Check sheet for the modelled part. Datum: model origin and axes. Units: mm. Round coordinates to 2 decimals unless told otherwise and drop trailing zeros. Loops run counter-clockwise (first coordinate to the right, second up) from the corner with the lowest first, then second, coordinate; pieces in that order, holes last. Notation, with made-up numbers: (7, 48) - (26, 48) arc R18 cw to (26, 56) - close; hole circle Ø2 at (26, 27). An arc over 180 degrees is marked (long way). Return JSON: item names as keys, results as strings.
from build123d import *

# Parameters (mm, degrees)
TOP_PLATE_SKETCH_PROFILE_R   = 3.175
TOP_PLATE_SKETCH_PROFILE_R_2 = 2.69875
TOP_PLATE_EXTRUDE_DEPTH      = 12.7


with BuildPart() as part:
    # Top Plate Sketch Profile → Top Plate Extrude (new body)
    with BuildSketch(Plane.XY.offset(114.3)):
        with BuildLine():
            Line((50.8, 44.45), (50.8, -44.45))
            ThreePointArc((50.8, -44.45), (48.940128061, -48.940128061), (44.45, -50.8))
            Line((44.45, -50.8), (-44.45, -50.8))
            ThreePointArc((-44.45, -50.8), (-48.940128061, -48.940128061), (-50.8, -44.45))
            Line((-50.8, -44.45), (-50.8, 44.45))
            ThreePointArc((-50.8, 44.45), (-48.940128061, 48.940128061), (-44.45, 50.8))
            Line((-44.45, 50.8), (44.45, 50.8))
            ThreePointArc((44.45, 50.8), (48.940128061, 48.940128061), (50.8, 44.45))
        make_face()
        with Locations((42.8625, 0)):
            Circle(TOP_PLATE_SKETCH_PROFILE_R, mode=Mode.SUBTRACT)
        with Locations((-42.8625, 0)):
            Circle(TOP_PLATE_SKETCH_PROFILE_R, mode=Mode.SUBTRACT)
        with Locations((-42.8625, 42.8625)):
            Circle(TOP_PLATE_SKETCH_PROFILE_R_2, mode=Mode.SUBTRACT)
        with Locations((42.8625, 42.8625)):
            Circle(TOP_PLATE_SKETCH_PROFILE_R_2, mode=Mode.SUBTRACT)
        with Locations((42.8625, -42.8625)):
            Circle(TOP_PLATE_SKETCH_PROFILE_R_2, mode=Mode.SUBTRACT)
        with Locations((-42.8625, -42.8625)):
            Circle(TOP_PLATE_SKETCH_PROFILE_R_2, mode=Mode.SUBTRACT)
    extrude(amount=-TOP_PLATE_EXTRUDE_DEPTH)


solid = part.part
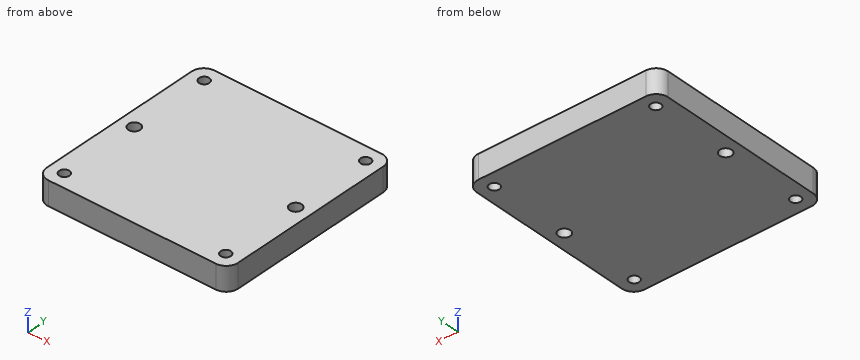
Q1. Sectioned sample at A-A (y = 0). Enter the section's corners in (x, z), plus the area to 3 significant figures.
Answer key:
{"outline": "(-50.8, 101.6) - (-46.04, 101.6) - (-46.04, 114.3) - (-50.8, 114.3) - close; (-39.69, 101.6) - (39.69, 101.6) - (39.69, 114.3) - (-39.69, 114.3) - close; (46.04, 101.6) - (50.8, 101.6) - (50.8, 114.3) - (46.04, 114.3) - close", "area": "1,130 mm²"}
Q2. Depth check by flat-ended pin: P1, Ø10, axis at x = 42.86, y = 0, coming from the +Z side. Enter the tip coordinate at first touch or a pass-through.
Answer key:
{"P1": "stops at z = 114.3"}
Q3. Sectioned sample at B-B (z = 106). State how many separate pieces and enclosed holes the cut face has, plus the area to 3 significant figures.
Answer key:
{"separate pieces": "1", "enclosed holes": "6", "area": "10,100 mm²"}
Q4. Scan lines: probe 1 along Y at (x, z) = (43, 109.75); probe 2 along Y at (x, z) = (42, 106.75); probe 3 along X at (y, z) = (42, 107.75). Record each from-to range of solid material in increasing order. Write a range as [from, to].
Answer key:
{"probe 1": "y = [-50.8, -45.56], [-40.17, -3.17], [3.17, 40.17], [45.56, 50.8]", "probe 2": "y = [-50.8, -45.42], [-40.31, -3.06], [3.06, 40.31], [45.42, 50.8]", "probe 3": "x = [-50.8, -45.42], [-40.31, 40.31], [45.42, 50.8]"}
